```python
from build123d import *

# Parameters (mm, degrees)
MAIN_SKETCH_W                          = 37
MAIN_SKETCH_H                          = 76
MAIN_EXTRUSION_DEPTH                   = 3
BOARD_FIX_SKETCH_R                     = 4
BOARD_FIX_SKETCH_R_2                   = 1.35
BOARD_FIX_DEPTH                        = 2
JACK_FIX_SKETCH_W                      = 4
JACK_FIX_SKETCH_H                      = 15
JACK_FIX_DEPTH                         = 15
JACK_FIX_HOLE_SKETCH_R                 = 3.75
JACK_FIX_HOLE_DEPTH                    = 21.75
JACK_FIX_REINFORCEMENT_EXTRUSION_DEPTH = 15


with BuildPart() as part:
    # Main-Sketch → Main-Extrusion (new body)
    with BuildSketch(Plane.XY):
        with Locations((18.5, 38)):
            Rectangle(MAIN_SKETCH_W, MAIN_SKETCH_H)
    extrude(amount=MAIN_EXTRUSION_DEPTH)

    # Board-Fix-Sketch → Board-Fix (add)
    with BuildSketch(Plane.XY.offset(3)):
        with Locations((3.75, 3)):
            Circle(BOARD_FIX_SKETCH_R)
        with Locations((3.75, 3)):
            Circle(BOARD_FIX_SKETCH_R_2, mode=Mode.SUBTRACT)
        with Locations((33.25, 3)):
            Circle(BOARD_FIX_SKETCH_R)
        with Locations((33.25, 3)):
            Circle(BOARD_FIX_SKETCH_R_2, mode=Mode.SUBTRACT)
        with Locations((33.25, 53.5)):
            Circle(BOARD_FIX_SKETCH_R)
        with Locations((33.25, 53.5)):
            Circle(BOARD_FIX_SKETCH_R_2, mode=Mode.SUBTRACT)
        with Locations((3.75, 53.5)):
            Circle(BOARD_FIX_SKETCH_R)
        with Locations((3.75, 53.5)):
            Circle(BOARD_FIX_SKETCH_R_2, mode=Mode.SUBTRACT)
    extrude(amount=BOARD_FIX_DEPTH)

    # Jack-Fix-Sketch → Jack-Fix (add)
    with BuildSketch(Plane.XY.offset(3)):
        with Locations((18.5, 68.5)):
            Rectangle(JACK_FIX_SKETCH_W, JACK_FIX_SKETCH_H)
    extrude(amount=JACK_FIX_DEPTH)

    # Jack-Fix-Hole-Sketch → Jack-Fix-Hole (cut, through all)
    with BuildSketch(Plane(origin=(20.5, 0, 0), x_dir=(0, 0, -1), z_dir=(1, 0, 0))):
        with Locations((-12, 68.5)):
            Circle(JACK_FIX_HOLE_SKETCH_R)
    extrude(amount=-JACK_FIX_HOLE_DEPTH, mode=Mode.SUBTRACT)

    # Jack-Fix-Reinforcement-Sketch → Jack-Fix-Reinforcement-Extrusion (add)
    with BuildSketch(Plane(origin=(0, 61, 0), x_dir=(-1, 0, 0), z_dir=(0, -1, 0))):
        Polygon((-22.5, -3), (-14.5, -3), (-16.5, -6), (-20.5, -6), align=None)
    extrude(amount=-JACK_FIX_REINFORCEMENT_EXTRUSION_DEPTH)


solid = part.part
```
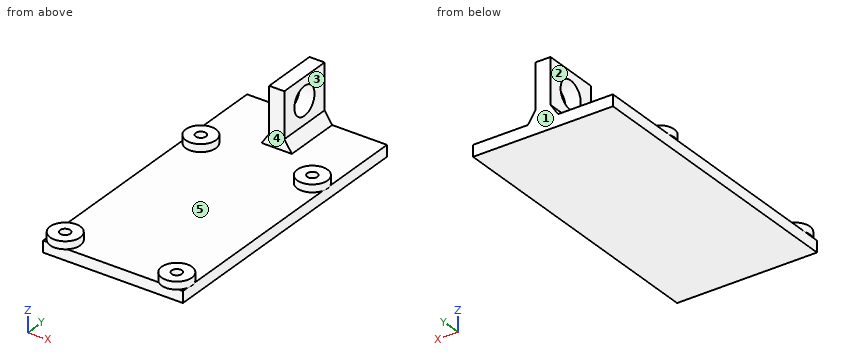
Source: CAD feature listing. Evaluate the final solid. Frame: model axes, mm. Face numbers are marked on the shaded views. A direction names the side the tool comes from. Round coordinates to 2 decimals unless told otherwise and drop trailing zeros. Order: outer loops, then holes, each group sorted by start corner. A loop starts at its lowest first (then second) coordinate and runs counter-clockwise, first axis right, second up. Notation, with made-up numbers: (76, -38.5) -> (91, -38.5) arc R10 cw to (91, -31.5) -> close; hole circle Ø10 at (-1.5, 9.5). An arc over 180 degrees is marked (long way). Use CSV: the item, a comma, the result in double quotes.
(1) Access query for the marked faces 1 and 2. Directions: +Z, -Z, +X, -X, +Y, -Y. A direction counts if a zero-diameter tool reaches every point of the face in a straight line with its end or side. Return the directions, or none.
Report:
face 1,"+Z, -Z, +X, -X, +Y"
face 2,"+Z, -X, +Y, -Y"
(2) Section A-A on y = 68.5. Return the cut outline in (x, z), and give its area (3 significant figures).
Report:
outline,"(0, 0) -> (37, 0) -> (37, 3) -> (22.5, 3) -> (20.5, 6) -> (20.5, 8.25) -> (16.5, 8.25) -> (16.5, 6) -> (14.5, 3) -> (0, 3) -> close; (16.5, 15.75) -> (20.5, 15.75) -> (20.5, 18) -> (16.5, 18) -> close"
area,"147 mm^2"
(3) First-contact query: pin 1 Ø2.5 at (x, y) = (33, 52) entering from +Z; pin 2 Ø6 at (y, z) = (65, 11.5) entering from +X; pin 3 Ø2 at (x, y) = (3.5, 3) entering from +Z; pin 4 Ø1.5 at (x, y) = (22, 47.5) entering from -Z. Flat tips, straight axial feed; report the tip coordinate or a pass-through.
Report:
pin 1,"z = 5"
pin 2,"x = 20.5"
pin 3,"z = 3"
pin 4,"z = 0"
(4) Section D-D on y = 3. Return the cut outline in (x, z), and give its area (3 significant figures).
Report:
outline,"(-0.25, 3) -> (0, 3) -> (0, 0) -> (37, 0) -> (37, 3) -> (37.25, 3) -> (37.25, 5) -> (34.6, 5) -> (34.6, 3) -> (31.9, 3) -> (31.9, 5) -> (29.25, 5) -> (29.25, 3) -> (7.75, 3) -> (7.75, 5) -> (5.1, 5) -> (5.1, 3) -> (2.4, 3) -> (2.4, 5) -> (-0.25, 5) -> close"
area,"132 mm^2"
(5) Section B-B on x = 19.5. Return the cut outline in (y, z).
Report:
outline,"(0, 0) -> (76, 0) -> (76, 18) -> (61, 18) -> (61, 3) -> (0, 3) -> close; hole circle Ø7.5 at (68.5, 12)"
(6) Section C-C on z = 12. Return the cut outline in (x, y), and give its area (3 significant figures).
Report:
outline,"(16.5, 61) -> (20.5, 61) -> (20.5, 64.75) -> (16.5, 64.75) -> close; (16.5, 72.25) -> (20.5, 72.25) -> (20.5, 76) -> (16.5, 76) -> close"
area,"30.0 mm^2"
(7) Pull-direction query (Y, two-part tool) for the marked faces 3, 4 and 5; classes: +Y half, -Y half, draft (parallel to the pull), parting line (faces both ways), or undercut.
Report:
face 3,"draft"
face 4,"-Y half"
face 5,"undercut"
(8) Ray query, L1, parallel to Y at x = 3.75, z = 3.5; L2, parallel to Y at x = 19.3, z = 12; L3, parallel to X at y = 62.5, z = 2.25. Return the intervals inside material, ascending.
Report:
L1,"-1 to 1.65, 4.35 to 7, 49.5 to 52.15, 54.85 to 57.5"
L2,"61 to 64.75, 72.25 to 76"
L3,"0 to 37"
